from build123d import *

# Parameters (mm, degrees)
SKETCH1_W           = 37.5
SKETCH1_H           = 42
BOSS_EXTRUDE1_DEPTH = 5
SKETCH2_W           = 37.5
SKETCH2_H           = 1
CUT_EXTRUDE1_DEPTH  = 3
SKETCH3_W           = 37.5
SKETCH3_H           = 1
CUT_EXTRUDE2_DEPTH  = 3
SKETCH4_W           = 10
SKETCH4_H           = 20
CUT_EXTRUDE3_DEPTH  = 1
FILLET1_R           = 10
FILLET2_R           = 10
SHELL1_START        = -16.25
SHELL1_DEPTH        = 32.5
SHELL1_2_DEPTH      = 8.75
SHELL1_START_2      = 7.5
SHELL1_3_DEPTH      = 8.75
SKETCH5_R           = 3
CUT_EXTRUDE4_DEPTH  = 2.5


# Read off the part's stored shape, not the designer's step: Shell1
with BuildPart() as part:
    # Sketch1 → Boss-Extrude1 (new body)
    with BuildSketch(Plane(origin=(0, 0, 0), x_dir=(1, 0, 0), z_dir=(0, 1, 0))):
        Rectangle(SKETCH1_W, SKETCH1_H)
    extrude(amount=BOSS_EXTRUDE1_DEPTH)

    # Sketch2 → Cut-Extrude1 (cut)
    with BuildSketch(Plane(origin=(0, 5, 0), x_dir=(1, 0, 0), z_dir=(0, 1, 0))):
        with Locations((0, -20.5)):
            Rectangle(SKETCH2_W, SKETCH2_H)
    extrude(amount=-CUT_EXTRUDE1_DEPTH, mode=Mode.SUBTRACT)

    # Sketch3 → Cut-Extrude2 (cut)
    with BuildSketch(Plane(origin=(0, 5, 0), x_dir=(1, 0, 0), z_dir=(0, 1, 0))):
        with Locations((0, 20.5)):
            Rectangle(SKETCH3_W, SKETCH3_H)
    extrude(amount=-CUT_EXTRUDE2_DEPTH, mode=Mode.SUBTRACT)

    # Sketch4 → Cut-Extrude3 (cut)
    with BuildSketch(Plane(origin=(0, 5, 0), x_dir=(1, 0, 0), z_dir=(0, 1, 0))):
        Rectangle(SKETCH4_W, SKETCH4_H)
    extrude(amount=-CUT_EXTRUDE3_DEPTH, mode=Mode.SUBTRACT)

    # Fillet1
    # the kernel refuses this fillet: 10 mm, written as the material it adds along each edge
    with BuildSketch(Plane(origin=(15.897247359, 4, -10), x_dir=(0, 1, 0), z_dir=(-1, 0, 0))) as fillet1_piece_1:
        with BuildLine():
            CenterArc((10, -4.358898944), FILLET1_R, 154.158067237, 25.841932763)
            Line((0, -4.358898944), (-0.2, -4.358898944))
            Line((-0.2, -4.358898944), (-0.2, 0))
            Line((-0.2, 0), (0, 0.2))
            ThreePointArc((0, 0.2), (0.5, 0.2), (0.82, 0.087177979))
            Line((0.82, 0.087177979), (1, 0))
        make_face()
    extrude(amount=31.794494718)

    # Fillet2
    # the kernel refuses this fillet: 10 mm, written as the material it adds along each edge
    with BuildSketch(Plane(origin=(-15.897247359, 4, 10), x_dir=(0, 0, -1), z_dir=(1, 0, 0))) as fillet2_piece_1:
        with BuildLine():
            CenterArc((4.358898944, 10), FILLET2_R, 244.158067237, 25.841932763)
            Line((0, 1), (-0.087177979, 0.82))
            ThreePointArc((-0.087177979, 0.82), (-0.2, 0.5), (-0.2, 0))
            Line((-0.2, 0), (0, -0.2))
            Line((0, -0.2), (4.358898944, -0.2))
            Line((4.358898944, -0.2), (4.358898944, 0))
        make_face()
    extrude(amount=31.794494718)

    # Shell1 outline → Shell1 (cut)
    with BuildSketch(Plane.YZ.offset(SHELL1_START)):
        with BuildLine():
            Line((0, -17.5), (2.5, -17.5))
            Line((2.5, -17.5), (2.5, -10.540080542))
            ThreePointArc((2.5, -10.540080542), (1.752551286, -8.141101056), (1.5, -5.641101056))
            Line((1.5, -5.641101056), (1.5, 5.641101056))
            ThreePointArc((1.5, 5.641101056), (1.752551286, 8.141101056), (2.5, 10.540080542))
            Line((2.5, 10.540080542), (2.5, 17.5))
            Line((2.5, 17.5), (0, 17.5))
            Line((0, 17.5), (0, -17.5))
        make_face()
    extrude(amount=SHELL1_DEPTH, mode=Mode.SUBTRACT)

    # Shell1 2 outline → Shell1 2 (cut)
    with BuildSketch(Plane.YZ.offset(SHELL1_START)):
        with BuildLine():
            ThreePointArc((1.5, -5.641101056), (1.752551286, -8.141101056), (2.5, -10.540080542))
            Line((2.5, -10.540080542), (2.5, 10.540080542))
            ThreePointArc((2.5, 10.540080542), (1.752551286, 8.141101056), (1.5, 5.641101056))
            Line((1.5, 5.641101056), (1.5, -5.641101056))
        make_face()
    extrude(amount=SHELL1_2_DEPTH, mode=Mode.SUBTRACT)

    # Shell1 3 outline → Shell1 3 (cut)
    with BuildSketch(Plane.YZ.offset(SHELL1_START_2)):
        with BuildLine():
            ThreePointArc((1.5, -5.641101056), (1.752551286, -8.141101056), (2.5, -10.540080542))
            Line((2.5, -10.540080542), (2.5, 10.540080542))
            ThreePointArc((2.5, 10.540080542), (1.752551286, 8.141101056), (1.5, 5.641101056))
            Line((1.5, 5.641101056), (1.5, -5.641101056))
        make_face()
    extrude(amount=SHELL1_3_DEPTH, mode=Mode.SUBTRACT)

    # Sketch5 → Cut-Extrude4 (cut)
    with BuildSketch(Plane(origin=(0, 5, 0), x_dir=(1, 0, 0), z_dir=(0, 1, 0))):
        with Locations(Location((-12.220002529, -10, 0), (0, 0, 270))):
            Circle(SKETCH5_R)
        with Locations(Location((-12.220002529, 10, 0), (0, 0, 270))):
            Circle(SKETCH5_R)
        with Locations(Location((12.411971657, -10, 0), (0, 0, 270))):
            Circle(SKETCH5_R)
        with Locations(Location((12.411971657, 10, 0), (0, 0, 270))):
            Circle(SKETCH5_R)
    extrude(amount=-CUT_EXTRUDE4_DEPTH, mode=Mode.SUBTRACT)


solid = part.part
Geometry: final body of the model. Coordinates: model frame, mm. A direction names the side the tool comes from. Round coordinates to 2 decimals unless told otherwise and drop trailing zeros. Order: outer loops, then holes, each group sorted by start corner. A loop starts at its lowest first (then second) coordinate and runs counter-clockwise, first axis right, second up.
Q1. Access query for faces 1 (the face through (-11, 2.5, 0)), 2 (the face through (-5, 4.5, 0.1)), 3 (the face through (-0.3, 2, 20.5)). Directions: +Z, -Z, +X, -X, +Y, -Y. A direction counts if a zero-diameter tool reaches every point of the face in a straight line with its end or side. Return the directions, or none.
Result sheet:
face 1: -Y
face 2: +Y
face 3: +Z, +X, -X, +Y
Q2. Section D-D, the plane x = -3. Output: boundary loops of the cut face in (y, z), and give its area (3 significant figures).
Result sheet:
outline: (0, -21) - (2, -21) - (2, -20) - (5, -20) - (5, -10) arc R10 cw to (4, -5.64) - (4, 5.64) arc R10 cw to (5, 10) - (5, 20) - (2, 20) - (2, 21) - (0, 21) - (0, 17.5) - (2.5, 17.5) - (2.5, 10.54) arc R12.5 ccw to (1.5, 5.64) - (1.5, -5.64) arc R12.5 ccw to (2.5, -10.54) - (2.5, -17.5) - (0, -17.5) - close
area: 117 mm2
Q3. Section B-B, the plane x = -13. Output: boundary loops of the cut face in (y, z), and give its area (3 significant figures).
Result sheet:
outline: (0, -21) - (2, -21) - (2, -20) - (5, -20) - (5, -12.9) - (2.5, -12.9) - (2.5, -17.5) - (0, -17.5) - close; (0, 17.5) - (2.5, 17.5) - (2.5, 12.9) - (5, 12.9) - (5, 20) - (2, 20) - (2, 21) - (0, 21) - close; (2.5, -7.1) - (5, -7.1) - (5, 7.1) - (2.5, 7.1) - close
area: 87.5 mm2
Q4. Section A-A, the plane z = -4.5. Output: boundary loops of the cut face in (x, y).
Result sheet:
outline: (-18.75, 0) - (-16.25, 0) - (-16.25, 2.5) - (-7.5, 2.5) - (-7.5, 1.5) - (7.5, 1.5) - (7.5, 2.5) - (16.25, 2.5) - (16.25, 0) - (18.75, 0) - (18.75, 5) - (5, 5) - (5, 4) - (-5, 4) - (-5, 5) - (-18.75, 5) - close
Q5. Mould query, pull axis X, two halves, no side actions, for faces 4 (the face through (0.07, 4.26, -7.91)), 5 (the face through (-0.3, 2, -20.5)). Classes: released by +X, released by -X, zero draft, split by the parting line, or undercut.
Result sheet:
face 4: undercut
face 5: zero draft
Q6. Section C-C, the plane z = -12. Output: boundary loops of the cut face in (x, y), and give its area (3 significant figures).
Result sheet:
outline: (-18.75, 0) - (-16.25, 0) - (-16.25, 2.5) - (-14.46, 2.5) - (-14.46, 5) - (-18.75, 5) - close; (-9.98, 2.5) - (10.18, 2.5) - (10.18, 5) - (-9.98, 5) - close; (14.65, 2.5) - (16.25, 2.5) - (16.25, 0) - (18.75, 0) - (18.75, 5) - (14.65, 5) - close
area: 83.9 mm2
Q7. Material intervals for probe 1 along X at (y, z) = (3.55, -10); probe 2 along X at (y, z) = (2.65, 12.5); probe 3 along X at (y, z) = (2.25, 10), sorted ascending.
Result sheet:
probe 1: x = -18.75 to -15.22, -9.22 to 9.41, 15.41 to 18.75
probe 2: x = -18.75 to -13.88, -10.56 to 10.75, 14.07 to 18.75
probe 3: x = -18.75 to -16.25, 16.25 to 18.75
Q8. Pin query (flat end, axial travel): pin 1 (1 mm diameter, centred on x = -9, z = -2.5, fed in from -Y); pin 2 (1.5 mm diameter, centred on x = 2, z = 5, fed in from +Y); pin 3 (12.5 mm diameter, centred on x = 1, z = -0.5, fed in from -Y). Return the tip coordinate at first contact, or that it passes through.
Result sheet:
pin 1: stops at y = 2.5
pin 2: stops at y = 4
pin 3: stops at y = 1.5
